Here's how the part is built. I have some questions about the finished solid (model axes, mm). A direction names the side the tool comes from. Give positions to 0.01 mm unless a question says otherwise; leave off trailing zeros. Order: outer loops, then holes, each group sorted by start corner. A loop starts at its lowest first (then second) coordinate and runs counter-clockwise, first axis right, second up. Notation, with made-up numbers: (57, 65) - (77, 65) arc R28 cw to (77, 95) - close; hole circle Ø5 at (-39, 66.5). An arc over 180 degrees is marked (long way). One line per question, with ' | ' between items.
from build123d import *

# Parameters (mm, degrees)
F0_R     = 15
F1_DEPTH = 120
F2_W     = 16.33073
F2_H     = 8.984623
F3_DEPTH = 9.652


with BuildPart() as f1:
    # F0 (on Top) → F1 (new body)
    with BuildSketch(Plane.XY):
        Circle(F0_R)
    extrude(amount=-F1_DEPTH)

    # F2 (on Top) → F3 (cut)
    with BuildSketch(Plane.XY):
        with Locations((0, 4.492311)):
            Rectangle(F2_W, F2_H)
    extrude(amount=-F3_DEPTH, mode=Mode.SUBTRACT)


solid = f1.part
1) I want a section at D-D (x = 5.75). List the corners of the cut face in (y, z) for me.
Model answer:
outline: (-13.85, -120) - (13.85, -120) - (13.85, 0) - (8.98, 0) - (8.98, -9.65) - (0, -9.65) - (0, 0) - (-13.85, 0) - close
2) I want a section at C-C (y = 13). List the corners of the cut face in (x, z) for me.
Model answer:
outline: (-7.48, -120) - (7.48, -120) - (7.48, 0) - (-7.48, 0) - close
3) Please list where these lines run through material, in increasing order: L1, parallel to Z at x = 5.25, y = 3; L2, parallel to X at y = 0.5, z = -71.5; L3, parallel to Y at x = 7, z = -8.
Model answer:
L1: z = -120 to -9.65 | L2: x = -14.99 to 14.99 | L3: y = -13.27 to 0, 8.98 to 13.27
4) On a 3-axis mill with a long thin cutter (end or side, diameter ignored), from which of +Z, -Z, +X, -X, +Y, -Y can I reach the whole of each face in a straight line? I mean faces 4 (the face through (0, -3, 0)), 5 (the face through (0, 5, -9.652)). Say none if no direction works.
Model answer:
face 4: +Z, +X, -X, +Y, -Y | face 5: +Z
5) I want a section at B-B (z = -96). List the corners of the cut face in (x, y) for me.
Model answer:
outline: circle Ø30 at (0, 0)
6) Thinking about a two-plate mould opening in X: for faces 1 (the face through (0, 0, -120)), 2 (the face through (0, 0, -5)), 3 (the face through (-14.985, 0.66, -59.16)), which applies, +X half, -X half, draft (parallel to the pull), parting line (faces both ways), or undercut?
Model answer:
face 1: draft | face 2: undercut | face 3: parting line
7) I'm going to push flat-ended pins straight in: P1, Ø4.5, axis at y = 4, z = -6, coming from the -X side; P2, Ø1, axis at x = -12, z = -95.5, coming from the -Y side; P3, Ø5, axis at y = -7, z = -77, coming from the +X side. Where does each tip first touch, or does it pass through?
Model answer:
P1: stops at x = -14.9 | P2: stops at y = -9.63 | P3: stops at x = 14.31
8) I want a section at A-A (x = 0). List the corners of the cut face in (y, z) for me, plus the area to 3 significant figures.
Model answer:
outline: (-15, -120) - (15, -120) - (15, 0) - (8.98, 0) - (8.98, -9.65) - (0, -9.65) - (0, 0) - (-15, 0) - close | area: 3,510 mm2
